Read the model definition and answer for the solid it produces. Units are mm, in the model's axes. A direction names the side the tool comes from. Coordinates: 2 decimals unless noted, no trailing zeros. Write each loop counter-clockwise with the first axis right and the second up, starting at its lowest first coordinate (ties: lowest second). Pieces come first, ordered by that corner, then holes. Notation, with made-up numbers: (-7, -17.5) -> (3, -17.5) arc R12 ccw to (3, -11.5) -> close; hole circle Ø3 at (57, 71). An arc over 180 degrees is marked (long way). Use CSV: the item, a comma, the result in double quotes.
from build123d import *

# Parameters (mm, degrees)
SKETCH1_W           = 50
SKETCH1_H           = 50
BOSS_EXTRUDE1_DEPTH = 50
CHAMFER1_SIZE       = 1.5
SKETCH2_W           = 1
SKETCH2_H           = 7
BOSS_EXTRUDE2_DEPTH = 7
SKETCH3_W           = 1.8
SKETCH3_H           = 1.8
CUT_EXTRUDE1_DEPTH  = 91.006944177


with BuildPart() as part:
    # Sketch1 → Boss-Extrude1 (new body)
    with BuildSketch(Plane.XY):
        with Locations((25, 25)):
            Rectangle(SKETCH1_W, SKETCH1_H)
    extrude(amount=BOSS_EXTRUDE1_DEPTH)

    # Chamfer1
    chamfer1_edges = [part.edges().sort_by_distance(p)[0] for p in [
        (50, 25, 50),
        (25, 50, 50),
        (0, 25, 50),
        (25, 50, 0),
        (50, 25, 0),
        (25, 0, 0),
        (0, 25, 0),
        (25, 0, 50),
        (0, 50, 25),
        (50, 50, 25),
        (50, 0, 25),
        (0, 0, 25),
    ]]
    chamfer(chamfer1_edges, length=CHAMFER1_SIZE)

    # Sketch2 → Boss-Extrude2 (add)
    with BuildSketch(Plane.XY.offset(50)):
        with Locations((48, 25)):
            Rectangle(SKETCH2_W, SKETCH2_H)
    extrude(amount=BOSS_EXTRUDE2_DEPTH)

    # Sketch3 → Cut-Extrude1 (cut, through all)
    with BuildSketch(Plane(origin=(48.5, 0, 0), x_dir=(0, 0, -1), z_dir=(1, 0, 0))):
        with Locations((-53.6, 25)):
            Rectangle(SKETCH3_W, SKETCH3_H)
    extrude(amount=-CUT_EXTRUDE1_DEPTH, mode=Mode.SUBTRACT)


solid = part.part
1. A cutting plane is placed at C-C (z = 51.5). Give the vertices of the cut face in (x, y), and give its area (3 significant figures).
Solutions:
outline,"(47.5, 21.5) -> (48.5, 21.5) -> (48.5, 28.5) -> (47.5, 28.5) -> close"
area,"7.00 mm^2"
2. A cutting plane is placed at A-A (y = 45.5). Give the vertices of the cut face in (x, z), and give its area (3 significant figures).
Solutions:
outline,"(0, 1.5) -> (1.5, 0) -> (48.5, 0) -> (50, 1.5) -> (50, 48.5) -> (48.5, 50) -> (1.5, 50) -> (0, 48.5) -> close"
area,"2,500 mm^2"
3. A tool of negligible diameter and unlimited length cuts with its end or side. For faces 4 (the flat face through (47.5, 25, 52)), 5 (the flat face through (48.5, 25, 52)), 6 (the flat face through (24.7, 0.8, 49.3)), from which of +Z, -Z, +X, -X, +Y, -Y can it reach the whole face along a straight path? Write none if from no direction.
Solutions:
face 4,"+Z, -X, +Y, -Y"
face 5,"+Z, +X, +Y, -Y"
face 6,"+Z, +X, -X, -Y"
4. Each of these flat-tipped pins is pushed along its axis until it touches: pin 1 Ø0.5 at (x, z) = (48, 53.5) entering from -Y; pin 2 Ø3.5 at (y, z) = (23.5, 55) entering from +X; pin 3 Ø2 at (y, z) = (26.5, 54) entering from -X. Where does it stop, or does it pass through?
Solutions:
pin 1,"stops at y = 21.5"
pin 2,"stops at x = 48.5"
pin 3,"stops at x = 47.5"
5. Find the intervals of material crossed by line 1 along Z through (x, y) = (25, 29); line 2 along Y through (x, z) = (42.5, 49), in increasing order.
Solutions:
line 1,"z = 0 to 50"
line 2,"y = 0.5 to 49.5"
6. For a pull along Z with two mould halves and no side action, classify faces 1 (the flat face through (24.7, 0.8, 0.7)), 2 (the flat face through (24.7, 49.2, 49.3)), 3 (the flat face through (49.2, 49.3, 24.7)) as pulls with the +Z half, pulls with the -Z half, needs draft (parallel to the pull), parting line crosses it, or undercut.
Solutions:
face 1,"pulls with the -Z half"
face 2,"pulls with the +Z half"
face 3,"needs draft"
